CAD build for the part. Positions are in the model's coordinates, mm. A direction names the side the tool comes from. Give positions to 0.01 mm unless a question says otherwise; leave off trailing zeros. Loops run counter-clockwise (first coordinate to the right, second up) from the corner with the lowest first, then second, coordinate; pieces in that order, holes last. Notation, with made-up numbers: M 54.5,0 L 101.5,0 A25 ccw 101.5,18 Z; hole C 21,59 d1. An arc over 180 degrees is marked long. Answer as CSV lines item,"result".
```python
from build123d import *

# Parameters (mm, degrees)
SKETCH1_W           = 34
SKETCH1_H           = 58
BOSS_EXTRUDE1_DEPTH = 13
CUT_EXTRUDE1_DEPTH  = 2.7
SKETCH5_R           = 4.3
CUT_EXTRUDE2_DEPTH  = 36.158071619
CUT_EXTRUDE3_DEPTH  = 45
CUT_EXTRUDE4_DEPTH  = 37.041642582
SKETCH9_R           = 1.1
CUT_EXTRUDE5_DEPTH  = 13
SKETCH10_R          = 2.1
CUT_EXTRUDE6_DEPTH  = 3
SKETCH12_W          = 34
SKETCH12_H          = 5
CUT_EXTRUDE7_DEPTH  = 15


with BuildPart() as part:
    # Sketch1 → Boss-Extrude1 (new body)
    with BuildSketch(Plane(origin=(0, 0, 0), x_dir=(1, 0, 0), z_dir=(0, 1, 0))):
        Rectangle(SKETCH1_W, SKETCH1_H)
    extrude(amount=BOSS_EXTRUDE1_DEPTH)

    # Sketch3 → Cut-Revolve1 (revolve, cut)
    with BuildSketch(Plane(origin=(0, 0, 0), x_dir=(0, 0, -1), z_dir=(1, 0, 0)), mode=Mode.PRIVATE) as cut_revolve1_sk:
        Polygon((-17, 13), (-12.05, 13), (-12.05, 2.6), (-10.6, 2.6), (-10.6, 0), (-17, 0), align=None)
    revolve(cut_revolve1_sk.sketch.rotate(Axis((0, 13, 17), (0, -1, 0)), 180), axis=Axis((0, 13, 17), (0, -1, 0)), mode=Mode.SUBTRACT)

    # Sketch4 → Cut-Extrude1 (cut)
    with BuildSketch(Plane.XZ):
        Polygon((3.70947548, -5.425), (7.418950959, 1), (3.70947548, 7.425), (-3.70947548, 7.425), (-7.418950959, 1), (-3.70947548, -5.425), align=None)
    extrude(amount=-CUT_EXTRUDE1_DEPTH, mode=Mode.SUBTRACT)

    # Sketch5 → Cut-Extrude2 (cut, through all)
    with BuildSketch(Plane.XZ.offset(-2.7)):
        with Locations(Location((0, 1, 0), (0, 0, 270))):
            Circle(SKETCH5_R)
    extrude(amount=-CUT_EXTRUDE2_DEPTH, mode=Mode.SUBTRACT)

    # Sketch6 → Cut-Extrude3 (cut)
    with BuildSketch(Plane(origin=(0, 0, -29), x_dir=(-1, 0, 0), z_dir=(0, 0, -1))):
        Polygon((-17, 6), (-14, 6), (-14, 9), (-6.699377385, 9), (-8.8, 6), (-8.8, 0), (-17, 0), align=None)
        Polygon((8.8, 0), (17, 0), (17, 6), (14, 6), (14, 9), (6.699377385, 9), (8.8, 6), align=None)
    extrude(amount=-CUT_EXTRUDE3_DEPTH, mode=Mode.SUBTRACT)

    # Sketch7 → Cut-Extrude4 (cut, through all)
    with BuildSketch(Plane(origin=(0, 13, 0), x_dir=(1, 0, 0), z_dir=(0, 1, 0))):
        with BuildLine():
            Line((17, -29), (17, -18.253317763))
            ThreePointArc((17, -18.253317763), (10.05598304, -26.088042865), (1.4e-08, -29))
            Line((1.4e-08, -29), (17, -29))
        make_face()
        with BuildLine():
            Line((-17, -29), (1.4e-08, -29))
            ThreePointArc((1.4e-08, -29), (-10.055983028, -26.088042873), (-17, -18.253317763))
            Line((-17, -18.253317763), (-17, -29))
        make_face()
    extrude(amount=-CUT_EXTRUDE4_DEPTH, mode=Mode.SUBTRACT)

    # Sketch11 → Cut-Revolve2 (revolve, cut)
    with BuildSketch(Plane(origin=(0, 0, 0), x_dir=(0, 0, -1), z_dir=(1, 0, 0))):
        Polygon((15, 0), (15, 13), (19.95, 13), (19.95, 2.6), (21.4, 2.6), (21.4, 0), align=None)
    revolve(axis=Axis((0, 0, -15), (0, 1, 0)), mode=Mode.SUBTRACT)

    # Sketch9 → Cut-Extrude5 (cut)
    with BuildSketch(Plane.XZ):
        with Locations(Location((0, -7, 0), (0, 0, 270))):
            Circle(SKETCH9_R)
        with Locations(Location((0, 9, 0), (0, 0, 270))):
            Circle(SKETCH9_R)
    extrude(amount=-CUT_EXTRUDE5_DEPTH, mode=Mode.SUBTRACT)

    # Sketch10 → Cut-Extrude6 (cut)
    with BuildSketch(Plane(origin=(0, 13, 0), x_dir=(1, 0, 0), z_dir=(0, 1, 0))):
        with Locations(Location((0, 7, 0), (0, 0, 270))):
            Circle(SKETCH10_R)
        with Locations(Location((0, -9, 0), (0, 0, 270))):
            Circle(SKETCH10_R)
    extrude(amount=-CUT_EXTRUDE6_DEPTH, mode=Mode.SUBTRACT)

    # Sketch12 → Cut-Extrude7 (cut)
    with BuildSketch(Plane(origin=(0, 13, 0), x_dir=(1, 0, 0), z_dir=(0, 1, 0))):
        with Locations((0, 26.5)):
            Rectangle(SKETCH12_W, SKETCH12_H)
    extrude(amount=-CUT_EXTRUDE7_DEPTH, mode=Mode.SUBTRACT)


solid = part.part
```
Q1. Cut at D-D (y = 12). Write the cut outline in (x, z), and give its area (3 significant figures).
Solution:
outline,"M -17,-24 L 17,-24 L 17,18.25 A18.82 ccw -17,18.25 Z; hole C 0,-15 d9.9; hole C 0,17 d9.9; hole C 0,1 d8.6; hole C 0,-7 d4.2; hole C 0,9 d4.2"
area,"1,460 mm²"
Q2. Mould opens along Y. For faces 1 (the flat face through (-1, 10, -6)), 2 (the flat face through (10, 9, -4)), 3 (the flat face through (5.538, 1.331, -2.257)) say: released by +Y, released by -Y, zero draft, split by the parting line, or undercut.
Solution:
face 1,"released by +Y"
face 2,"undercut"
face 3,"zero draft"
Q3. Cut at C-C (z = -15). Write the cut outline in (x, y), and give its area (3 significant figures).
Solution:
outline,"M -17,6 L -14,6 L -14,9 L -6.7,9 L -8.8,6 L -8.8,0 L -6.4,0 L -6.4,2.6 L -4.95,2.6 L -4.95,13 L -17,13 Z; M 4.95,2.6 L 6.4,2.6 L 6.4,0 L 8.8,0 L 8.8,6 L 6.7,9 L 14,9 L 14,6 L 17,6 L 17,13 L 4.95,13 Z"
area,"170 mm²"
Q4. Wall check: line 1 (X direction, y = 7.5, z = -19); line 2 (Z direction, x = -0.5, y = 9.5); line 3 (X direction, y = 2.5, z = -7). Give the ranges that are in metal, low to high. Write a range as [from, to].
Solution:
line 1,"x = [-17, -14], [-7.75, -2.92], [2.92, 7.75], [14, 17]"
line 2,"z = [-24, -19.92], [-10.08, -7.98], [-6.02, -3.27], [5.27, 8.02], [9.98, 12.08], [21.92, 28.99]"
line 3,"x = [-8.8, -1.1], [1.1, 8.8]"
Q5. Cut at A-A (z = 9). Write the cut outline in (x, y).
Solution:
outline,"M -17,6 L -14,6 L -14,9 L -6.7,9 L -8.8,6 L -8.8,0 L -1.1,0 L -1.1,10 L -2.1,10 L -2.1,13 L -17,13 Z; M 1.1,0 L 8.8,0 L 8.8,6 L 6.7,9 L 14,9 L 14,6 L 17,6 L 17,13 L 2.1,13 L 2.1,10 L 1.1,10 Z"
Q6. Pin check, flat tips, straight feed: P1, Ø1, axis at x = -0.5, z = -11.5, coming from the +Y side; P2, Ø3, axis at x = 0, z = 9, coming from the +Y side; P3, Ø3.5, axis at x = 15, z = -13, coming from the -Y side; P4, Ø3, axis at x = 3, y = 8, coming from the +Z side. Stop position of each tip, or through.
Solution:
P1,"passes through"
P2,"stops at y = 10"
P3,"stops at y = 6"
P4,"stops at z = 28.94"
Q7. Cut at B-B (y = 4.25). Write the cut outline in (x, z).
Solution:
outline,"M -17,16 L -8.8,16 L -8.8,-24 L 8.8,-24 L 8.8,16 L 17,16 L 17,18.25 A18.82 ccw -17,18.25 Z; hole C 0,-15 d9.9; hole C 0,17 d9.9; hole C 0,1 d8.6; hole C 0,-7 d2.2; hole C 0,9 d2.2"
Q8. Which spindle directions (+Z, -Z, +X, -X, +Y, -Y) get a long thin tool onto all of the face, cutting with end or side? Do faces 4 (the flat face through (-8.8, 3, -4)), 5 (the flat face through (-14, 7, -4)), 6 (the cylindrical face through (0.09, 11.52, 6.9)), 7 (the flat face through (-5.538, 1.331, 4.257)). Say none if no direction does.
Solution:
face 4,"-Z, -X, -Y"
face 5,"-Z, -Y"
face 6,"+Y"
face 7,"-Y"
